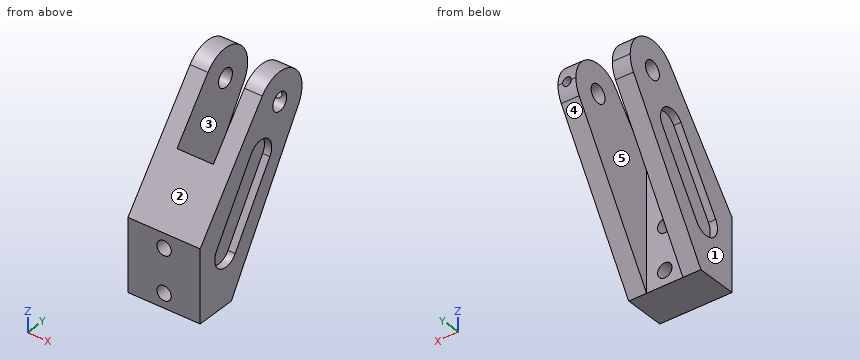
```python
from build123d import *

# Parameters (mm, degrees)
F0_R      = 1.5875
F1_DEPTH  = 12.7
F2_R      = 1.27
F3_DEPTH  = 25.4
F5_DEPTH  = 32.767
F7_R      = 0.762
F8_DEPTH  = 5.08
F10_DEPTH = 1.27
F12_DEPTH = 1.27


with BuildPart() as f1:
    # F0 (on Right) → F1 (new body)
    with BuildSketch(Plane.YZ):
        with BuildLine():
            ThreePointArc((22.5126934436, 25.0233725308), (23.0743428543, 26.3023762602), (23.2664, 27.686))
            ThreePointArc((23.2664, 27.686), (19.8428720781, 32.4883432046), (14.1866754903, 30.817869066))
            Line((14.1866754903, 30.817869066), (0, 12.7))
            Line((0, 12.7), (0, 0))
            Line((0, 0), (7.112, 0))
            Line((7.112, 0), (22.5126934436, 25.0233725308))
        make_face()
        with Locations((18.1864, 27.686)):
            Circle(F0_R, mode=Mode.SUBTRACT)
    extrude(amount=-F1_DEPTH)

    # F2 (on face) → F3 (cut)
    with BuildSketch(Plane.XZ):
        with Locations((-6.35, 10.16)):
            Circle(F2_R)
        with Locations((-6.35, 2.54)):
            Circle(F2_R)
    extrude(amount=-F3_DEPTH, mode=Mode.SUBTRACT)

    # F4 (on face) → F5 (cut, through all)
    with BuildSketch(Plane(origin=(0, 0, 0), x_dir=(1, 0, 0), z_dir=(0, 0, -1))):
        Polygon((-5.5372, -7.112), (-7.1628, -7.112), (-9.5504, -7.112), (-9.5504, -9.4996), (-9.5504, -27.9279650633), (-3.1496, -27.9279650633), (-3.1496, -9.4996), (-3.1496, -7.112), align=None)
    extrude(amount=-F5_DEPTH, mode=Mode.SUBTRACT)

    # F7 (on plane+point) → F8 (cut)
    with BuildSketch(Plane.XZ.offset(-23.2664)):
        with Locations((-1.5849518823, 27.6825465262)):
            Circle(F7_R)
    extrude(amount=F8_DEPTH, mode=Mode.SUBTRACT)

    # F9 (on face) → F10 (cut)
    with BuildSketch(Plane.YZ):
        with BuildLine():
            Line((11.667870953, 22.4236173585), (3.743070953, 10.3332173585))
            ThreePointArc((3.743070953, 10.3332173585), (4.4749826415, 6.816470953), (7.991729047, 7.5483826415))
            Line((7.991729047, 7.5483826415), (15.916529047, 19.6387826415))
            ThreePointArc((15.916529047, 19.6387826415), (15.1846173585, 23.155529047), (11.667870953, 22.4236173585))
        make_face()
    extrude(amount=-F10_DEPTH, mode=Mode.SUBTRACT)

    # F11 (on face) → F12 (cut)
    with BuildSketch(Plane(origin=(-12.7, 0, 0), x_dir=(0, -1, 0), z_dir=(-1, 0, 0))):
        with BuildLine():
            Line((-15.916529047, 19.6387826415), (-7.991729047, 7.5483826415))
            ThreePointArc((-7.991729047, 7.5483826415), (-4.4749826415, 6.816470953), (-3.743070953, 10.3332173585))
            Line((-3.743070953, 10.3332173585), (-11.667870953, 22.4236173585))
            ThreePointArc((-11.667870953, 22.4236173585), (-15.1846173585, 23.155529047), (-15.916529047, 19.6387826415))
        make_face()
    extrude(amount=-F12_DEPTH, mode=Mode.SUBTRACT)


solid = f1.part
```
Check sheet for the modelled part. Datum: model origin and axes. Units: mm. Face numbers are marked on the shaded views. A direction names the side the tool comes from. Round coordinates to 2 decimals unless told otherwise and drop trailing zeros. Order: outer loops, then holes, each group sorted by start corner. A loop starts at its lowest first (then second) coordinate and runs counter-clockwise, first axis right, second up. Notation, with made-up numbers: (-12, 3.25) -> (38, 3.25) arc R20 ccw to (38, 35.25) -> close; hole circle Ø11 at (-15, 86). An arc over 180 degrees is marked (long way). One line per item, written item: value. Start each with the question number.
Q1. Cross-section at B-B (y = 21.75). Record the boundary of the cut face in (x, z), and give its area (3 significant figures).
Q2. Cross-section at D-D (y = 5.25). Record the boundary of the cut face in (x, z), and give its area (3 significant figures).
Q3. Gauge pin test, flat ends, axial feed: pin 1 Ø3.5 at (x, z) = (-6.35, 10.16) entering from +Y; pin 2 Ø5 at (x, y) = (-6, 2.5) entering from +Z; pin 3 Ø3 at (y, z) = (18.19, 27.69) entering from -X; pin 4 Ø7 at (x, z) = (-6.5, 6) entering from +Y. Record the tip position at first contact, or that the pin passes through.
Q4. Thickness scan on line 1 (X direction, y = 19.75, z = 29); line 2 (Z direction, x = -6.35, y = 4); line 3 (Z direction, x = -6.35, y = 5). Record the ranges inside material, lowest first.
Q5. Mould release check, pull along X, two halves, no side actions. Record for the marked faces 1, 2 and 3: pulls with the +X half, pulls with the -X half, needs draft (parallel to the pull), parting line crosses it, or undercut.
Q6. Cross-section at A-A (x = -6.35). Record the boundary of the cut face in (y, z).
Q7. Cross-section at C-C (z = 2.54). Record the boundary of the cut face in (x, y), and give its area (3 significant figures).
Q8. Set-up check for the marked faces 4 and 5: record each of +Z, -Z, +X, -X, +Y, -Y from which the full face is reachable in a straight line by a thin tool's end or side.
Completed:
1. outline: (-12.7, 23.78) -> (-9.55, 23.78) -> (-9.55, 31.31) -> (-12.7, 31.31) -> close; (-3.15, 23.78) -> (0, 23.78) -> (0, 31.31) -> (-3.15, 31.31) -> close; hole circle Ø1.52 at (-1.58, 27.68)
1. area: 45.6 mm²
2. outline: (-12.7, 0) -> (0, 0) -> (0, 6.48) -> (-1.27, 6.48) -> (-1.27, 12.63) -> (0, 12.63) -> (0, 19.4) -> (-12.7, 19.4) -> (-12.7, 12.63) -> (-11.43, 12.63) -> (-11.43, 6.48) -> (-12.7, 6.48) -> close; hole circle Ø2.54 at (-6.35, 2.54); hole circle Ø2.54 at (-6.35, 10.16)
2. area: 221 mm²
3. pin 1: stops at y = 7.11
3. pin 2: stops at z = 19.09
3. pin 3: passes through
3. pin 4: stops at y = 11.86
4. line 1: x = -12.7 to -9.55, -3.15 to 0
4. line 2: z = 0 to 1.27, 3.81 to 8.89, 11.43 to 17.81
4. line 3: z = 0 to 1.27, 3.81 to 8.89, 11.43 to 19.09
5. face 1: pulls with the -X half
5. face 2: needs draft
5. face 3: undercut
6. outline: (0, 0) -> (7.11, 0) -> (7.11, 1.27) -> (0, 1.27) -> close; (0, 3.81) -> (7.11, 3.81) -> (7.11, 8.89) -> (0, 8.89) -> close; (0, 11.43) -> (7.11, 11.43) -> (7.11, 21.78) -> (0, 12.7) -> close
7. outline: (-12.7, 0) -> (-7.62, 0) -> (-7.62, 7.11) -> (-9.55, 7.11) -> (-9.55, 8.68) -> (-12.7, 8.68) -> close; (-5.08, 0) -> (0, 0) -> (0, 8.68) -> (-3.15, 8.68) -> (-3.15, 7.11) -> (-5.08, 7.11) -> close
7. area: 82.1 mm²
8. face 4: -Z, +X, -X, +Y
8. face 5: +Z, -Z, +Y
